Check sheet for the modelled part. Datum: model origin and axes. Units: mm. Face numbers are marked on the shaded views. A direction names the side the tool comes from. Round coordinates to 2 decimals unless told otherwise and drop trailing zeros. Write each loop counter-clockwise with the first axis right and the second up, starting at its lowest first coordinate (ties: lowest second). Pieces come first, ordered by that corner, then holes. Notation, with made-up numbers: (48.5, 15) -> (84.5, 15) arc R4 ccw to (84.5, 19) -> close; hole circle Ø8 at (-10.5, -0.5). An arc over 180 degrees is marked (long way). Write item = value, one per line.
Autodesk Inventor part; units mm, degrees
ref_plane "YZ Plane" through (0, 0, 0) normal (1, 0, 0) x (0, 1, 0)
ref_plane "XZ Plane" through (0, 0, 0) normal (0, 1, 0) x (-1, 0, 0)
ref_plane "XY Plane" through (0, 0, 0) normal (0, 0, 1) x (1, 0, 0)
sketch "Sketch1" plane through (0, 0, 0) normal (0, 1, 0) x (-1, 0, 0)
  line L0 (12.25, 22.5) -> (-12.25, 22.5)
  line L1 (-12.25, 22.5) -> (-12.25, -22.5)
  line L2 (-12.25, -22.5) -> (12.25, -22.5)
  line L3 (12.25, -22.5) -> (12.25, 22.5)
  point P0 (0, 0)
  point P1 (12.25, 0)
  point P2 (0, 22.5)
  dimension "d0" = 24.5
  dimension "d1" = 45
extrude "Extrusion1" add sketch "Sketch1" along normal blind 1.95
sketch "Sketch2" plane through (0, 1.95, 0) normal (0, 1, 0) x (1, 0, 0)
  line L0 (-10, 1.25) -> (10, 1.25)
  line L1 (10, 1.25) -> (10, -17.25)
  line L2 (10, -17.25) -> (-10, -17.25)
  line L3 (-10, -17.25) -> (-10, 1.25)
  line L4 (-12.25, -22.5) -> (12.25, -22.5)
  line L5 (12.25, -22.5) -> (12.25, 22.5)
  line L6 (12.25, 22.5) -> (-12.25, 22.5)
  line L7 (-12.25, 22.5) -> (-12.25, -22.5)
  line L8 (-7, -17.25) -> (7, -17.25)
  line L9 (7, -17.25) -> (7, -22.5)
  line L10 (7, -22.5) -> (-7, -22.5)
  line L11 (-7, -22.5) -> (-7, -17.25)
  line L12 (-12.25, -22.5) -> (12.25, -22.5)
  point P0 (0, 0)
  dimension "d4" = 2.25
  dimension "d5" = 20
  dimension "d6" = 2.25
  dimension "d7" = 5.25
  dimension "d8" = 5.25
  dimension "d9" = 14
  dimension "d10" = 5.25
  dimension "d11" = 18.5
extrude "Extrusion2" cut sketch "Sketch2" against normal up to surface (1.95 mm away) contours L0 L1 L2 L3 | L2 L9 L4 L11
sketch "Sketch3" plane through (0, 1.95, 0) normal (0, 1, 0) x (1, 0, 0)
  line L0 (-7, -22.5) -> (-7, -17.25)
  line L1 (-7, -17.25) -> (-10, -17.25)
  line L2 (-10, -17.25) -> (-10, 1.25)
  line L3 (-10, 1.25) -> (10, 1.25)
  line L4 (10, 1.25) -> (10, -17.25)
  line L5 (10, -17.25) -> (7, -17.25)
  line L6 (7, -17.25) -> (7, -22.5)
  line L7 (7, -22.5) -> (12.25, -22.5)
  line L8 (12.25, -22.5) -> (12.25, 22.5)
  line L9 (12.25, 22.5) -> (-12.25, 22.5)
  line L10 (-12.25, 22.5) -> (-12.25, -22.5)
  line L11 (-12.25, -22.5) -> (-7, -22.5)
  point P0 (0, 0)
  point P1 (-10.25, -20.305)
  point P2 (10.25, -20.305)
  dimension "d14" = 20.5
  dimension "d15" = 2
  dimension "d16" = 2.195
  dimension "d17" = 2
hole "Hole1" at (-10.25, 1.95, 20.305) at (10.25, 1.95, 20.305) direction (0, -1, 0) diameter 2.4 end through all
sketch "Sketch4" plane through (0, 1.95, 0) normal (0, 1, 0) x (1, 0, 0)
  circle A0 centre (-10.25, -20.305) radius 1.2
  circle A1 centre (10.25, -20.305) radius 1.2
  line L0 (-7, -22.5) -> (-7, -17.25)
  line L1 (-7, -17.25) -> (-10, -17.25)
  line L2 (-10, -17.25) -> (-10, 1.25)
  line L3 (-10, 1.25) -> (10, 1.25)
  line L4 (10, 1.25) -> (10, -17.25)
  line L5 (10, -17.25) -> (7, -17.25)
  line L6 (7, -17.25) -> (7, -22.5)
  line L7 (7, -22.5) -> (12.25, -22.5)
  line L8 (12.25, -22.5) -> (12.25, 22.5)
  line L9 (12.25, 22.5) -> (-12.25, 22.5)
  line L10 (-12.25, 22.5) -> (-12.25, -22.5)
  line L11 (-12.25, -22.5) -> (-7, -22.5)
  point P0 (0, 0)
  point P1 (-10.25, 4.15)
  point P2 (10.25, 4.15)
  dimension "d25" = 20.5
  dimension "d26" = 26.65
  dimension "d27" = 2
  dimension "d28" = 2
hole "Hole2" at (-10.25, 1.95, -4.15) at (10.25, 1.95, -4.15) direction (0, -1, 0) diameter 2.4 end through all
fillet "Fillet1" radius 0.5 2 edges at (7, 0.975, 17.25) (-7, 0.975, 17.25)
sketch "Sketch5" plane through (0, 1.95, 0) normal (0, 1, 0) x (1, 0, 0)
  circle A0 centre (-10.25, 4.15) radius 1.2
  circle A1 centre (10.25, 4.15) radius 1.2
  circle A2 centre (-10.25, -20.305) radius 1.2
  circle A3 centre (10.25, -20.305) radius 1.2
  arc A4 (-7, -17.75) -> (-7.5, -17.25) centre (-7.5, -17.75) ccw
  line L0 (-7.5, -17.25) -> (-10, -17.25)
  line L1 (-10, -17.25) -> (-10, 1.25)
  line L2 (-10, 1.25) -> (10, 1.25)
  line L3 (10, 1.25) -> (10, -17.25)
  line L4 (10, -17.25) -> (7.5, -17.25)
  arc A5 (7.5, -17.25) -> (7, -17.75) centre (7.5, -17.75) ccw
  line L5 (7, -17.75) -> (7, -22.5)
  line L6 (7, -22.5) -> (12.25, -22.5)
  line L7 (12.25, -22.5) -> (12.25, 22.5)
  line L8 (12.25, 22.5) -> (-12.25, 22.5)
  line L9 (-12.25, 22.5) -> (-12.25, -22.5)
  line L10 (-12.25, -22.5) -> (-7, -22.5)
  line L11 (-7, -22.5) -> (-7, -17.75)
  line L12 (-12.25, 22.5) -> (-12.25, -22.5)
  line L13 (12.25, -22.5) -> (12.25, 22.5)
  line L14 (-12.25, -22.5) -> (12.25, -22.5)
  line L15 (12.25, -22.5) -> (12.25, -4.5)
  line L16 (12.25, -4.5) -> (10, -4.5)
  line L17 (-12.25, -4.5) -> (-12.25, -22.5)
  line L18 (-10, -4.5) -> (-12.25, -4.5)
  line L19 (10, -4.5) -> (-10, -4.5)
  point P0 (0, 0)
  dimension "d37" = 18
extrude "Extrusion3" add sketch "Sketch5" along normal blind 5 contours L11 L10 L9 L18 L1 L0 A4 | A4 L0 L1 L19 L3 L4 A5 L5 L14 L11 | L5 A5 L4 L3 L16 L7 L6 | L18 L9 L8 L7 L16 L3 L2 L1
equation "\"d4\" = d6"
equation "\"d8\" = d10"
properties part number "servotest"
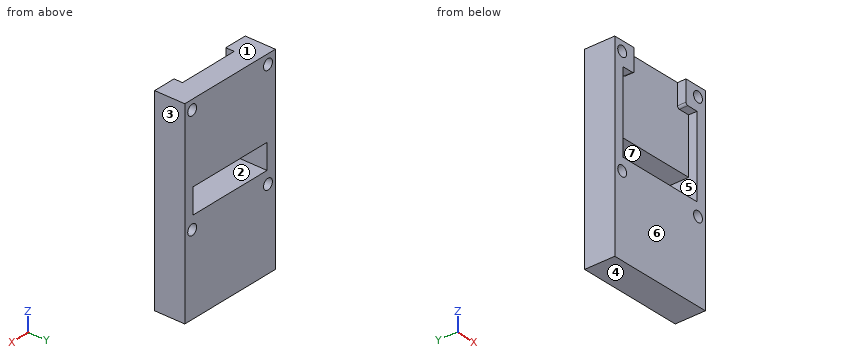
(1) Release check for a two-part mould opening along Z. For the marked faces 1, 2, 3 and 4 record: pulls with the +Z half, pulls with the -Z half, needs draft (parallel to the pull), parting line crosses it, or undercut.
Worked answers:
face_1 = pulls with the +Z half
face_2 = undercut
face_3 = needs draft
face_4 = pulls with the -Z half
(2) Sectioned sample at D-D on y = 3.5. Enter the section's corners in (x, z) (3 decimals).
Worked answers:
outline = (-12.25, -22.5) -> (12.25, -22.5) -> (12.25, 22.5) -> (-12.25, 22.5) -> close; hole circle Ø2.4 at (-10.25, -4.15); hole circle Ø2.4 at (-10.25, 20.305); hole (-10, -1.25) -> (10, -1.25) -> (10, 4.5) -> (-10, 4.5) -> close; hole circle Ø2.4 at (10.25, -4.15); hole circle Ø2.4 at (10.25, 20.305)
(3) Sectioned sample at C-C on y = 1.25. Enter the section's corners in (x, z) (3 decimals).
Worked answers:
outline = (-12.25, -22.5) -> (12.25, -22.5) -> (12.25, 22.5) -> (7, 22.5) -> (7, 17.75) arc R0.5 ccw to (7.5, 17.25) -> (10, 17.25) -> (10, -1.25) -> (-10, -1.25) -> (-10, 17.25) -> (-7.5, 17.25) arc R0.5 ccw to (-7, 17.75) -> (-7, 22.5) -> (-12.25, 22.5) -> close; hole circle Ø2.4 at (-10.25, -4.15); hole circle Ø2.4 at (-10.25, 20.305); hole circle Ø2.4 at (10.25, -4.15); hole circle Ø2.4 at (10.25, 20.305)
(4) Material ranges on L1, parallel to Z at x = -10.25, y = 3.5 (3 decimals); L2, parallel to X at y = 2, z = -4.15; L3, parallel to Z at x = -6.25, y = 4.25, recorded low to high. Write a range as [from, to].
Worked answers:
L1 = [-22.5, -5.35], [-2.95, 19.105], [21.505, 22.5]
L2 = [-12.25, -11.45], [-9.05, 9.05], [11.45, 12.25]
L3 = [-22.5, -1.25], [4.5, 22.5]
(5) Sectioned sample at B-B on z = 18.5. Enter the section's corners in (x, y), then the cut area to 3 significant figures.
Worked answers:
outline = (-12.25, 0) -> (-7, 0) -> (-7, 1.95) -> (7, 1.95) -> (7, 0) -> (12.25, 0) -> (12.25, 6.95) -> (-12.25, 6.95) -> close
area = 143 mm²
(6) Sectioned sample at A-A on z = 3. Enter the section's corners in (x, y), then the cut area to 3 significant figures.
Worked answers:
outline = (-12.25, 0) -> (-10, 0) -> (-10, 6.95) -> (-12.25, 6.95) -> close; (10, 0) -> (12.25, 0) -> (12.25, 6.95) -> (10, 6.95) -> close
area = 31.3 mm²
(7) Access from +Z, -Z, +X, -X, +Y, -Y to the whole of each face (thin tool, end or side, straight path). Record for the marked faces 5, 6 and 7.
Worked answers:
face_5 = -Y
face_6 = +Z, -Z, +X, -X, -Y
face_7 = +Y, -Y
(8) Go/stop test with flat-tipped pins: P1, Ø1.9, axis at x = -10.25, z = 20.305, coming from the +Y side; P2, Ø8, axis at x = -3, z = 11.5, coming from the -Y side. Record where each tip stops, or that it passes through.
Worked answers:
P1 = through
P2 = 1.95
